from build123d import *

# Parameters (mm, degrees)
FILLET1_R       = 0.1
FILLET2_R       = 0.3
HEX_2_DEPTH     = 1.3
THDSCHPAT_COUNT = 13
THDSCHPAT_PITCH = 0.5


with BuildPart() as part:
    # BodySke → Base-Revolve (revolve)
    with BuildSketch(Plane.XY, mode=Mode.PRIVATE) as base_revolve_sk:
        Polygon((0, 0), (0, 2.75), (3, 2.75), (3, 1.5), (10.7195, 1.5), (11, 1.2195), (11, 0), align=None)
    revolve(base_revolve_sk.sketch.rotate(Axis((-31.75, 0, 0), (1, 0, 0)), 90), axis=Axis((-31.75, 0, 0), (1, 0, 0)))  # turned: the seam where the file's is

    # Fillet1
    fillet1_edges = [part.edges().sort_by_distance(p)[0] for p in [
        (3, 0, -1.5),
    ]]
    fillet(fillet1_edges, radius=FILLET1_R)

    # Fillet2
    fillet2_edges = [part.edges().sort_by_distance(p)[0] for p in [
        (0, 0, -2.75),
    ]]
    fillet(fillet2_edges, radius=FILLET2_R)

    # Sketch2 → Hex-PreBroach (revolve, cut)
    with BuildSketch(Plane.XY, mode=Mode.PRIVATE) as hex_prebroach_sk:
        Polygon((0, 1.26), (1.3, 1.26), (2.027461339, 0), (0, 0), align=None)
    revolve(hex_prebroach_sk.sketch.rotate(Axis((0, 0, 0), (1, 0, 0)), 90), axis=Axis((0, 0, 0), (1, 0, 0)), mode=Mode.SUBTRACT)  # turned: the seam where the file's is

    # Sketch3 → Hex 2 (cut)
    with BuildSketch(Plane(origin=(0, 0, 0), x_dir=(0, 0.5, 0.866025404), z_dir=(-1, 0, 0))):
        Polygon((0.727461339, 1.26), (-0.727461339, 1.26), (-1.454922678, 0), (-0.727461339, -1.26), (0.727461339, -1.26), (1.454922678, 0), align=None)
    extrude(amount=-HEX_2_DEPTH, mode=Mode.SUBTRACT)

    # ThdSchSke → ThreadSchematic (revolve, cut)
    with BuildSketch(Plane.XY, mode=Mode.PRIVATE) as threadschematic_sk:
        Polygon((4.5, -1.2195), (4.303591786, -1.5), (4.303591786, -1.875), (4.696408214, -1.875), (4.696408214, -1.5), align=None)
    threadschematic = revolve(threadschematic_sk.sketch.rotate(Axis((-3.175, 0, 0), (1, 0, 0)), 270), axis=Axis((-3.175, 0, 0), (1, 0, 0)), mode=Mode.SUBTRACT)  # turned: the seam where the file's is

    # ThdSchPat: ThreadSchematic ×13
    with Locations(*[(i * THDSCHPAT_PITCH, 0, 0) for i in range(1, THDSCHPAT_COUNT)]):
        add(threadschematic, mode=Mode.SUBTRACT)


solid = part.part
Verification items for the finished model (mm, model axes). Give positions to 0.01 mm unless a question says otherwise; leave off trailing zeros. Write each loop counter-clockwise with the first axis right and the second up, starting at its lowest first coordinate (ties: lowest second). Pieces come first, ordered by that corner, then holes. Notation, with made-up numbers: M 6.5,5 L 27.5,5 A21 cw 27.5,18 Z; hole C -4.75,-36 d7. An arc over 180 degrees is marked long. Write item = value, one per line.
(1) Go/stop test with a flat-tipped pin: pin 1 Ø1 at (x, z) = (5, 1.5) entering from +Y. Record where the tip stops, or that it passes through.
Found:
pin_1 = 1.08
(2) Draft check along Y on faces 1 (the face through (0.641, -1.086, -0.639)), 2 (the face through (3.71, -0.45, 1.43)), 3 (the face through (0.641, 1.096, -0.621)). Enter one of: released by +Y, released by -Y, zero draft, split by the parting line, or undercut.
Found:
face_1 = undercut
face_2 = split by the parting line
face_3 = undercut
(3) Material ranges on line 1 (Z direction, x = 3.25, y = -0.35); line 2 (X direction, y = 0.6, z = 1.75); line 3 (X direction, y = 0, z = -0.7), recorded low to high.
Found:
line_1 = -1.46 to 1.46
line_2 = 0 to 3
line_3 = 1.62 to 11
(4) Sectioned sample at A-A (x = 2.5). Record the cut outline in (y, z), then the cut area to 3 significant figures.
Found:
outline = C 0,0 d5.5
area = 23.8 mm2
